from build123d import *

# Parameters (mm, degrees)
CROQUIS1_W              = 900
CROQUIS1_H              = 100
CROQUIS1_H_2            = 300
CROQUIS1_H_3            = 150
SALIENTE_EXTRUIR2_DEPTH = 25
CORTAR_EXTRUIR1_DEPTH   = 10
CROQUIS3_W              = 950
CROQUIS3_H              = 25
CORTAR_EXTRUIR2_DEPTH   = 850
CROQUIS4_W              = 200
CROQUIS4_H              = 25
SALIENTE_EXTRUIR3_DEPTH = 50
CROQUIS5_R              = 3.75
SALIENTE_EXTRUIR4_DEPTH = 10


with BuildPart() as part:
    # Croquis1 → Saliente-Extruir2 (new body)
    with BuildSketch(Plane(origin=(0, 0, 0), x_dir=(1, 0, 0), z_dir=(0, 1, 0))):
        Polygon((450, -475), (450, -575), (100, -575), (100, -600), (475, -600), (475, 600), (-475, 600), (-475, -600), (-100, -600), (-100, -575), (-450, -575), (-450, -475), align=None)
        with Locations((0, -325)):
            Rectangle(CROQUIS1_W, CROQUIS1_H, mode=Mode.SUBTRACT)
        with Locations((0, -25)):
            Rectangle(CROQUIS1_W, CROQUIS1_H_2, mode=Mode.SUBTRACT)
        with Locations((0, 350)):
            Rectangle(CROQUIS1_W, CROQUIS1_H_3, mode=Mode.SUBTRACT)
    extrude(amount=SALIENTE_EXTRUIR2_DEPTH)

    # Croquis2 → Cortar-Extruir1 (cut)
    with BuildSketch(Plane(origin=(-100, 0, 0), x_dir=(0, 0, -1), z_dir=(1, 0, 0))):
        with BuildLine():
            ThreePointArc((-583.75, 12.5), (-586.064937129, 15.964548247), (-590.151650429, 15.151650429))
            Line((-590.151650429, 15.151650429), (-584.848349571, 9.848349571))
            ThreePointArc((-584.848349571, 9.848349571), (-584.035451753, 11.064937129), (-583.75, 12.5))
        make_face()
        with BuildLine():
            Line((-584.848349571, 9.848349571), (-590.151650429, 15.151650429))
            ThreePointArc((-590.151650429, 15.151650429), (-590.151650429, 9.848349571), (-584.848349571, 9.848349571))
        make_face()
    extrude(amount=-CORTAR_EXTRUIR1_DEPTH, mode=Mode.SUBTRACT)

    # Croquis3 → Cortar-Extruir2 (cut)
    with BuildSketch(Plane(origin=(0, 0, -600), x_dir=(-1, 0, 0), z_dir=(0, 0, -1))):
        with Locations((0, 12.5)):
            Rectangle(CROQUIS3_W, CROQUIS3_H)
    extrude(amount=-CORTAR_EXTRUIR2_DEPTH, mode=Mode.SUBTRACT)

    # Croquis4 → Saliente-Extruir3 (add)
    with BuildSketch(Plane(origin=(0, 0, 250), x_dir=(-1, 0, 0), z_dir=(0, 0, -1))):
        with Locations((0, 12.5)):
            Rectangle(CROQUIS4_W, CROQUIS4_H)
    extrude(amount=SALIENTE_EXTRUIR3_DEPTH)

    # Croquis5 → Saliente-Extruir4 (add)
    with BuildSketch(Plane.ZY.offset(100)):
        with Locations((212.5, 12.5)):
            Circle(CROQUIS5_R)
    extrude(amount=SALIENTE_EXTRUIR4_DEPTH)


solid = part.part
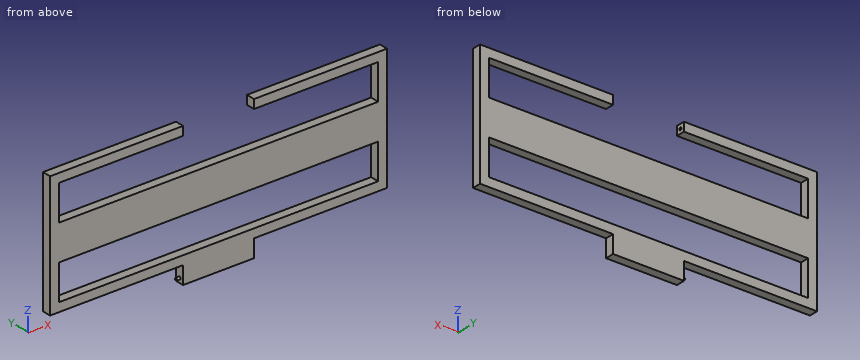
Input: part model. Units: mm. Frame: model coordinates. Round coordinates to 2 decimals unless told otherwise and drop trailing zeros. Write each loop counter-clockwise with the first axis right and the second up, starting at its lowest first coordinate (ties: lowest second). Pieces come first, ordered by that corner, then holes.
1) Contact query for flat-ended pins moving along their axis: P1, Ø12.5, axis at y = 13.5, z = 232, coming from the -X side; P2, Ø10, axis at x = 250.5, y = 14, coming from the -Z side; P3, Ø7.5, axis at y = 15.5, z = 226.5, coming from the +X side. Output: stop coordinate, or through.
2) Ray query, L1, parallel to Z at x = 375, y = 20.25; L2, parallel to X at y = 21.5, z = 353; L3, parallel to X at y = 3, z = 223. Return the intervals inside material, ascending.
3) Cut plane A-A (z = 510.5). Return the cut outline in (x, y), then the cut area to 3 significant figures.
4) Cut plane B-B (x = 409.5). Return the cut outline in (y, z), then the cut area to 3 significant figures.
Geometry says:
1. P1: stops at x = -100
1. P2: stops at z = 250
1. P3: stops at x = 100
2. L1: z = 250 to 275, 375 to 475, 575 to 600
2. L2: x = -475 to -450, 450 to 475
2. L3: x = -100 to 100
3. outline: (-475, 0) - (-450, 0) - (-450, 25) - (-475, 25) - close; (450, 0) - (475, 0) - (475, 25) - (450, 25) - close
3. area: 1,250 mm2
4. outline: (0, 250) - (25, 250) - (25, 275) - (0, 275) - close; (0, 375) - (25, 375) - (25, 475) - (0, 475) - close; (0, 575) - (25, 575) - (25, 600) - (0, 600) - close
4. area: 3,750 mm2
